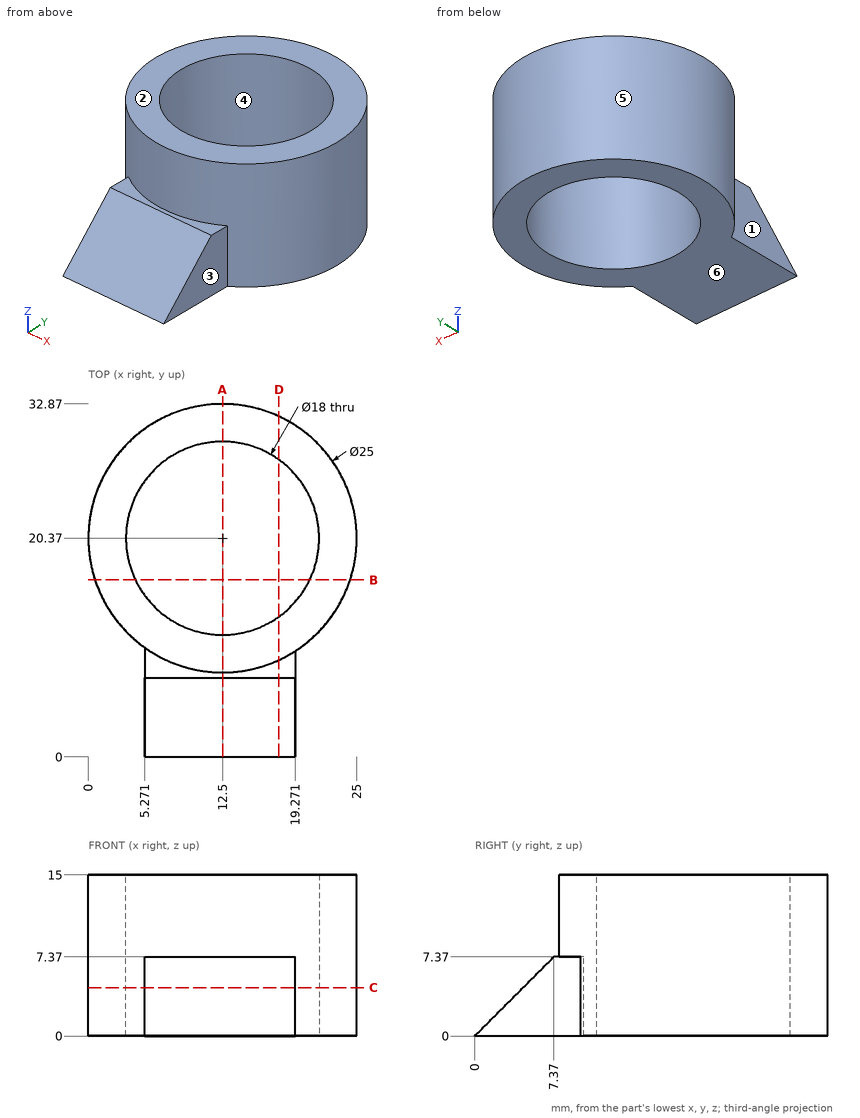
Can you work these out from the drawing? Everything is in mm from the part's minimum corner. A direction names the side the tool comes from. Round coordinates to 2 decimals unless told otherwise and drop trailing zeros. Write each loop counter-clockwise with the first axis right and the second up, starting at its lowest first coordinate (ties: lowest second). Pieces come first, ordered by that corner, then holes.
1. If we mould it in two halves opening along Y, with no side actions, what happens to the marked faces 4, 5 and 6? For each: released by +Y, released by -Y, zero draft, split by the parting line, or undercut.
2. Suppose I cut it at D-D (x = 17.75). List the corners of the cut face in (y, z) for me (1 decimal).
3. I need wall thicknesses on L1, parallel to Y at x = 12.5, z = 11.75; L2, parallel to Y at x = 17.25, z = 11.5 (1 decimal); L3, parallel to X at y = 15, z = 10.25. Which ranges of each line are inside material? Lowest first, please.
4. Suppose I cut it at B-B (y = 16.5). List the corners of the cut face in (x, z) for me (1 decimal), and give its area (3 significant figures).
5. Suppose I cut it at A-A (x = 12.5). List the corners of the cut face in (y, z) for me, and give its area (3 significant figures).
6. Will these pins go through, and if not, where does the flat tip stop? pin 1 Ø1 at (x, z) = (7, 8) entering from +Y; pin 2 Ø3.5 at (y, z) = (6, 4) entering from +X; pin 3 Ø1.5 at (x, z) = (17, 4) entering from -Y.
7. Suppose I cut it at C-C (z = 4.5). List the corners of the cut face in (x, y) for me.
8. For the marked faces 1, 2 and 3, which set-ups out of +Z, -Z, +X, -X, +Y, -Y let a thin tool reach every point of the face, with its end or its side?
Answer sheet:
1. face 4: undercut
1. face 5: split by the parting line
1. face 6: zero draft
2. outline: (0, 0) - (13.1, 0) - (13.1, 15) - (9, 15) - (9, 7.4) - (7.4, 7.4) - close; (27.7, 0) - (31.7, 0) - (31.7, 15) - (27.7, 15) - close
3. L1: y = 7.87 to 11.37, 29.37 to 32.87
3. L2: y = 8.8 to 12.7, 28 to 31.9
3. L3: x = 1.21 to 5.28, 19.72 to 23.79
4. outline: (0.6, 0) - (4.4, 0) - (4.4, 15) - (0.6, 15) - close; (20.6, 0) - (24.4, 0) - (24.4, 15) - (20.6, 15) - close
4. area: 113 mm2
5. outline: (0, 0) - (11.37, 0) - (11.37, 15) - (7.87, 15) - (7.87, 7.37) - (7.37, 7.37) - close; (29.37, 0) - (32.87, 0) - (32.87, 15) - (29.37, 15) - close
5. area: 136 mm2
6. pin 1: stops at y = 31.83
6. pin 2: stops at x = 19.27
6. pin 3: stops at y = 3.25
7. outline: (5.27, 4.5) - (19.27, 4.5) - (19.27, 9.86) arc R12.5 ccw (long way) to (5.27, 10.17) - close; hole circle Ø18 at (12.5, 20.37)
8. face 1: +Z, -Z, -X, -Y
8. face 2: +Z, +X, -X, +Y, -Y
8. face 3: +Z, -Z, +X, -Y
